Verification items for the finished model (mm, model axes). Coordinates: 2 decimals unless noted, no trailing zeros. Answer as a JSON object with one key per item and string values. Group by question number.
(1) Mould release check, pull along X, two halves, no side actions. Record for faces 1 (the face through (-2, -3.175, -1)), 2 (the face through (38.09, -0.04, -24.64)), 3 (the face through (-152.5, 0, 1)): released by +X, released by -X, zero draft, split by the parting line, or undercut.
(2) Gauge pin test, flat ends, axial feed: pin 1 Ø8 at (x, z) = (35.98, 25.98) entering from +Y (3 decimals); pin 2 Ø4 at (x, z) = (-135.98, 25.98) entering from -Y. Record the tip position at first contact, or that the pin passes through.
(3) Material ranges on line 1 (X direction, y = 1.2, z = 25.98); line 2 (Z direction, x = -135.98, y = 0.75); line 3 (X direction, y = -2.5, z = 9.5), recorded low to high.
from build123d import *

# Parameters (mm, degrees)
SKETCH1_W               = 305
SKETCH1_H               = 85
BOSS_EXTRUDE1_DEPTH     = 3.175
SKETCH4_R               = 2.5
CUT_EXTRUDE2_DEPTH      = 161.752389174
CUT_EXTRUDE3_DEPTH      = 159.438702658
CUT_EXTRUDE3_DEPTH_BACK = 159.438702658
SKETCH6_R               = 2.5
CUT_EXTRUDE4_DEPTH      = 159.438702658
CUT_EXTRUDE4_DEPTH_BACK = 159.438702658
SKETCH7_R               = 2.5


with BuildPart() as part:
    # Sketch1 → Boss-Extrude1 (new, symmetric)
    with BuildSketch(Plane(origin=(0, 0, 0), x_dir=(1, 0, 0), z_dir=(0, 1, 0))):
        Rectangle(SKETCH1_W, SKETCH1_H)
    extrude(amount=BOSS_EXTRUDE1_DEPTH, both=True)

    # Sketch4 → Cut-Extrude2 (cut, symmetric)
    with BuildSketch(Plane(origin=(-2.5, 0, 0), x_dir=(-1, 0, 0), z_dir=(0, -1, 0))):
        with Locations(Location((133.48, -25.98, 0), (0, 0, 90))):
            Circle(SKETCH4_R)
        with Locations(Location((133.48, 25.98, 0), (0, 0, 270))):
            Circle(SKETCH4_R)
    cut_extrude2 = extrude(amount=CUT_EXTRUDE2_DEPTH, both=True, mode=Mode.SUBTRACT)

    # Mirror2: Cut-Extrude2 across plane
    add(cut_extrude2.mirror(Plane.ZY.offset(50)), mode=Mode.SUBTRACT)

    # Sketch6 → Cut-Extrude3 (cut, two sides: drawn at the far end of the back side and taken through both)
    with BuildSketch(Plane(origin=(0, 3.175, 0), x_dir=(1, 0, 0), z_dir=(0, 1, 0)).offset(-CUT_EXTRUDE3_DEPTH_BACK)):
        with Locations(Location((-139.8, 8.75, 0), (0, 0, 270))):
            Circle(SKETCH6_R)
        with Locations(Location((-139.8, -8.75, 0), (0, 0, 270))):
            Circle(SKETCH6_R)
    extrude(amount=CUT_EXTRUDE3_DEPTH + CUT_EXTRUDE3_DEPTH_BACK, mode=Mode.SUBTRACT)

    # Sketch7 → Cut-Extrude4 (cut, two sides: drawn at the far end of the back side and taken through both)
    with BuildSketch(Plane.XZ.offset(3.175).offset(-CUT_EXTRUDE4_DEPTH_BACK)):
        with Locations(Location((139.6, -8.75, 0), (0, 0, 270))):
            Circle(SKETCH7_R)
        with Locations(Location((139.6, 8.75, 0), (0, 0, 270))):
            Circle(SKETCH7_R)
    extrude(amount=CUT_EXTRUDE4_DEPTH + CUT_EXTRUDE4_DEPTH_BACK, mode=Mode.SUBTRACT)


solid = part.part
Taken from the geometry:
{
 "1": {"face 1": "zero draft", "face 2": "undercut", "face 3": "released by -X"},
 "2": {"pin 1": "stops at y = 3.175", "pin 2": "passes through"},
 "3": {"line 1": "x = -152.5 to -138.48, -133.48 to 33.48, 38.48 to 152.5", "line 2": "z = -42.5 to -28.48, -23.48 to 23.48, 28.48 to 42.5", "line 3": "x = -152.5 to -142.18, -137.42 to 137.22, 141.98 to 152.5"}
}
